Check sheet for the drawn part. Datum: minimum x, y, z corner. Units: mm. A direction names the side the tool comes from. Give positions to 0.01 mm unless a question says otherwise; leave off trailing zeros. Write each loop counter-clockwise with the first axis right and the second up, starting at its lowest first coordinate (ties: lowest second). Pieces come first, ordered by that corner, then holes. Notation, with made-up numbers: M 51.5,57.5 L 80.5,57.5 A9 cw 80.5,74.5 Z; hole C 45.5,-31.75 d10. An arc over 180 degrees is marked long. Use CSV: the item, a comma, the result in double quotes. Start each with the question number.
1. Mould release check, pull along X, two halves, no side actions. Record for the marked faces 6, 7, 8 and 9: +X half, -X half, draft (parallel to the pull), parting line (faces both ways), or undercut.
2. Depth check by flat-ended pin: P1, Ø6, axis at y = 10, z = 94.5, coming from the -X side; P2, Ø6, axis at y = 13, z = 91, coming from the +X side; P3, Ø8, axis at x = 3, y = 12, coming from the -Z side. Enter the tip coordinate at first touch or a pass-through.
3. Cross-section at A-A, the plane y = 12.5. Enter the section's corners in (x, z), and give its area (4 significant figures).
4. Scan lines: line 1 (Y direction, x = 37, z = 88); line 2 (Z direction, x = 31, y = 26.25); line 3 (X direction, y = 27.75, z = 66.5). Record each from-to range of solid material in increasing order.
5. Cross-section at B-B, the plane z = 92. Enter the section's corners in (x, y).
6. Cross-section at C-C, the plane x = 7. Enter the section's corners in (y, z), and give its area (3 significant figures).
7. Access from +Z, -Z, +X, -X, +Y, -Y to the whole of each face (thin tool, end or side, straight path). Record for the marked faces 1, 2, 3, 4 and 5.
8. Cross-section at D-D, the plane z = 31.5. Enter the section's corners in (x, y), and give its area (3 significant figures).
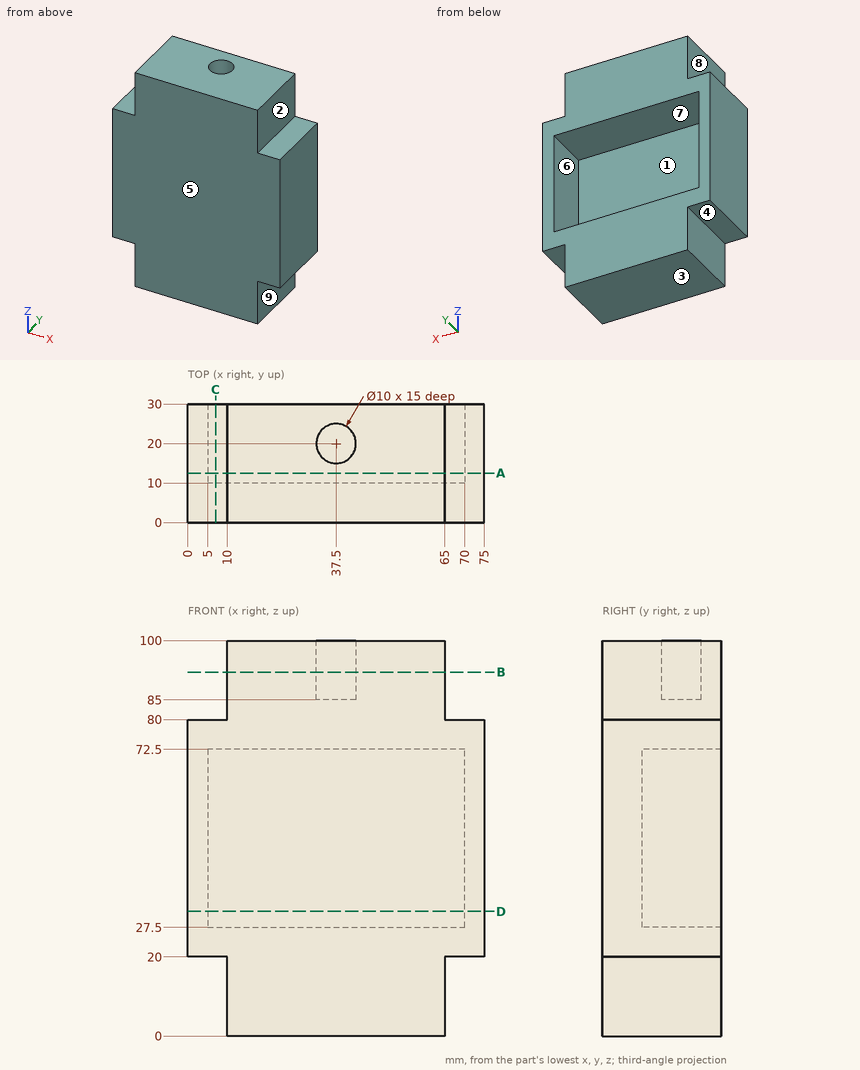
Worked answers:
1,face 6,"undercut"
1,face 7,"undercut"
1,face 8,"-X half"
1,face 9,"+X half"
2,P1,"stops at x = 10"
2,P2,"stops at x = 65"
2,P3,"stops at z = 20"
3,outline,"M 0,20 L 10,20 L 10,0 L 65,0 L 65,20 L 75,20 L 75,80 L 65,80 L 65,100 L 10,100 L 10,80 L 0,80 Z; hole M 5,27.5 L 70,27.5 L 70,72.5 L 5,72.5 Z"
3,area,"3,775 mm^2"
4,line 1,"y = 0 to 15.03, 24.97 to 30"
4,line 2,"z = 0 to 27.5, 72.5 to 100"
4,line 3,"x = 0 to 5, 70 to 75"
5,outline,"M 10,0 L 65,0 L 65,30 L 10,30 Z; hole C 37.5,20 d10"
6,outline,"M 0,20 L 30,20 L 30,27.5 L 10,27.5 L 10,72.5 L 30,72.5 L 30,80 L 0,80 Z"
6,area,"900 mm^2"
7,face 1,"+Y"
7,face 2,"+Z, +X, +Y, -Y"
7,face 3,"-Z, +X, -X, +Y, -Y"
7,face 4,"-Z, -X, +Y, -Y"
7,face 5,"+Z, -Z, +X, -X, -Y"
8,outline,"M 0,0 L 75,0 L 75,30 L 70,30 L 70,10 L 5,10 L 5,30 L 0,30 Z"
8,area,"950 mm^2"
